from build123d import *

# Parameters (mm, degrees)
SKETCH1_R           = 7.62
BOSS_EXTRUDE1_DEPTH = 2.54
BOSS_EXTRUDE2_DEPTH = 69.85


with BuildPart() as part:
    # Sketch1 → Boss-Extrude1 (new body)
    with BuildSketch(Plane(origin=(0, 0, 0), x_dir=(1, 0, 0), z_dir=(0, 1, 0))):
        with Locations(Location((0, 0, 0), (0, 0, 270))):
            Circle(SKETCH1_R)
    extrude(amount=BOSS_EXTRUDE1_DEPTH)

    # Sketch2 → Boss-Extrude2 (add)
    with BuildSketch(Plane(origin=(0, 2.54, 0), x_dir=(-1, 0, 0), z_dir=(0, 1, 0))):
        with BuildLine():
            Line((1.778, 4.445), (-1.778, 4.445))
            Line((-1.778, 4.445), (-1.778, 5.764527062))
            ThreePointArc((-1.778, 5.764527062), (-3.582266828, -4.853701745), (6.0325, 0))
            ThreePointArc((6.0325, 0), (4.853701745, 3.582266828), (1.778, 5.764527062))
            Line((1.778, 5.764527062), (1.778, 4.445))
        make_face()
    extrude(amount=BOSS_EXTRUDE2_DEPTH)


solid = part.part
The listing builds one solid part. Answer for the finished solid, in the listing's coordinates (mm). A direction names the side the tool comes from. Round coordinates to 2 decimals unless told otherwise and drop trailing zeros. Order: outer loops, then holes, each group sorted by start corner. A loop starts at its lowest first (then second) coordinate and runs counter-clockwise, first axis right, second up. Notation, with made-up numbers: M 34.25,15.25 L 48.25,15.25 A27 ccw 48.25,38.25 Z; hole C 61,24.25 d7. An arc over 180 degrees is marked long. Answer in a Markdown table with one row per item. Add a question column.
1) Determine the mould class of faces 3 (the face through (0, 37, 4.445)), 4 (the face through (7.555, 1.252, -0.992)), 5 (the face through (0, 0, 0)) for opening direction X: pulls with the +X half, pulls with the -X half, needs draft (parallel to the pull), parting line crosses it, or undercut.
2) The part is cut by section C-C on z = -1.25. Determine the outline of the cut face in (x, y).
3) The part is cut by section B-B on y = 24.5. Determine the outline of the cut face in (x, z) (1 decimal), plus the area to 3 significant figures.
4) The part is cut by section A-A on x = 0. Determine the outline of the cut face in (y, z) (1 decimal), plus the area to 3 significant figures.
5) Consider line 1 along Y through (x, z) = (-2.25, 5.75); line 2 along Z through (x, y) = (-0.25, 34) (3 decimals); line 3 along X through (y, z) = (39.5, 3.5). Determine where each line is inside the solid, lowest interval first. Write a range as from..to.
6) Flat-ended cylindrical pins translate along their axes: pin 1 Ø5 at (x, z) = (4.5, 2.5) entering from -Y; pin 2 Ø2 at (x, y) = (-2.5, 31) entering from -Z; pin 3 Ø4 at (y, z) = (45, 0) entering from -X; pin 4 Ø1.5 at (y, z) = (19, -4.5) entering from -X. Find the tip coordinate at first contact, or state that the pin passes through.
7) Which of the six approach directions +Z, -Z, +X, -X, +Y, -Y give full straight-line access (tool end or side, diameter ignored) to faces 1 (the face through (0, 72.39, 0)), 2 (the face through (1.778, 37, 5))?
Findings below:
| question | item | result |
|---|---|---|
| 1 | face 3 | undercut |
| 1 | face 4 | parting line crosses it |
| 1 | face 5 | needs draft |
| 2 | outline | M -7.52,0 L 7.52,0 L 7.52,2.54 L 5.9,2.54 L 5.9,72.39 L -5.9,72.39 L -5.9,2.54 L -7.52,2.54 Z |
| 3 | outline | M -1.8,4.4 L -1.8,5.8 A6 ccw long 1.8,5.8 L 1.8,4.4 Z |
| 3 | area | 109 mm² |
| 4 | outline | M 0,-7.6 L 2.5,-7.6 L 2.5,-6 L 72.4,-6 L 72.4,4.4 L 2.5,4.4 L 2.5,7.6 L 0,7.6 Z |
| 4 | area | 771 mm² |
| 5 | line 1 | y = 0..2.54 |
| 5 | line 2 | z = -6.027..4.445 |
| 5 | line 3 | x = -4.91..4.91 |
| 6 | pin 1 | stops at y = 0 |
| 6 | pin 2 | stops at z = -5.84 |
| 6 | pin 3 | stops at x = -6.03 |
| 6 | pin 4 | stops at x = -4.73 |
| 7 | face 1 | +Z, -Z, +X, -X, +Y |
| 7 | face 2 | +Z, +Y |
